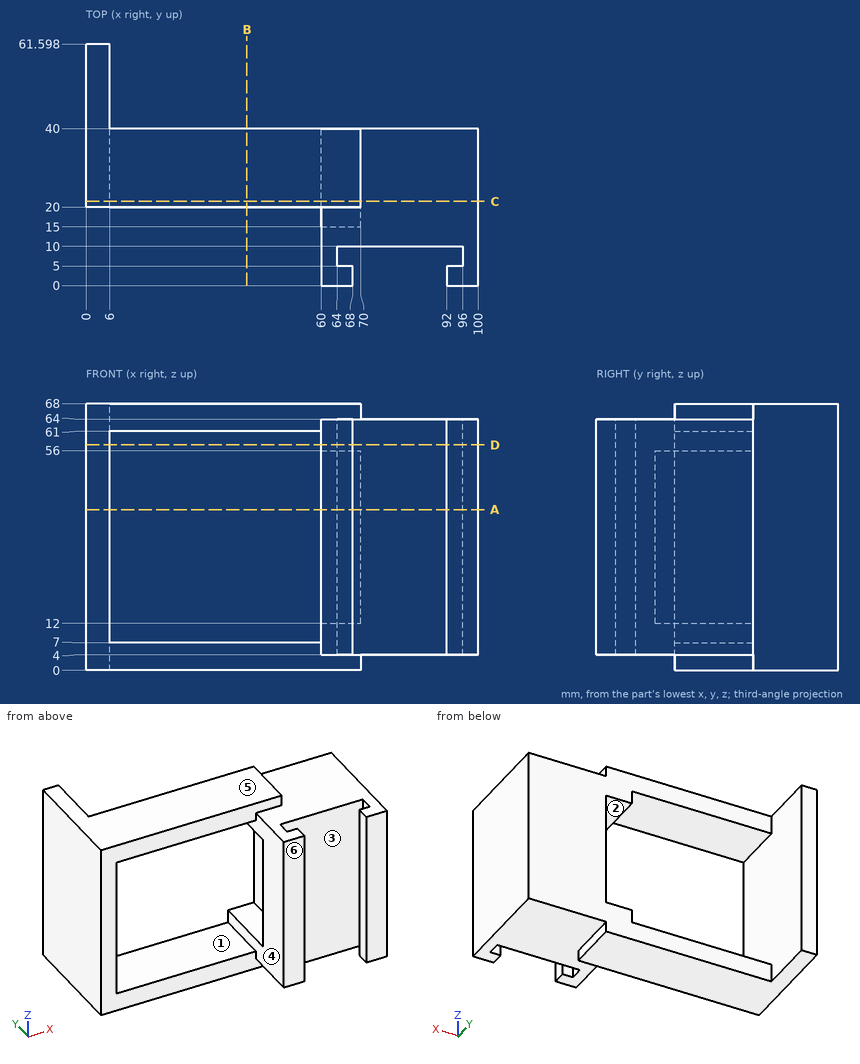
Source: three-view drawing plus pictorial views. Frame: mm from the lowest corner of the part. A direction names the side the tool comes from. Coordinates: 2 decimals unless noted, no trailing zeros. Order: outer loops, then holes, each group sorted by start corner. A loop starts at its lowest first (then second) coordinate and runs counter-clockwise, first axis right, second up. Notation, with made-up numbers: (47, 81.5) -> (93, 81.5) arc R21 ccw to (93, 100.5) -> close; hole circle Ø5 at (56, -39.5). An arc over 180 degrees is marked (long way). Write item = value, one per line.
(1) Pull-direction query (Z, two-part tool) for the marked faces 4, 5 and 6; classes: pulls with the +Z half, pulls with the -Z half, needs draft (parallel to the pull), parting line crosses it, or undercut.
Solved:
face_4 = undercut
face_5 = pulls with the +Z half
face_6 = needs draft
(2) Cut plane A-A on z = 41. Return loops of the section in (x, y), plus the area to 3 significant figures.
Solved:
outline = (0, 20) -> (6, 20) -> (6, 61.6) -> (0, 61.6) -> close; (60, 0) -> (68, 0) -> (68, 5) -> (64, 5) -> (64, 10) -> (96, 10) -> (96, 5) -> (92, 5) -> (92, 0) -> (100, 0) -> (100, 40) -> (70, 40) -> (70, 15) -> (60, 15) -> close
area = 1,320 mm²
(3) Pin query (flat end, axial travel): pin 1 Ø10 at (x, z) = (14, 7) entering from -Y; pin 2 Ø1.2 at (x, z) = (65.5, 42.5) entering from +Y; pin 3 Ø1.5 at (y, z) = (8, 41) entering from -X; pin 4 Ø20.5 at (x, z) = (34.5, 49.5) entering from +Y. Return the tip coordinate at first contact, or that it passes through.
Solved:
pin_1 = 20
pin_2 = 15
pin_3 = 60
pin_4 = through
(4) Access query for the marked faces 1, 2 and 3. Directions: +Z, -Z, +X, -X, +Y, -Y. A direction counts if a zero-diameter tool reaches every point of the face in a straight line with its end or side. Return the directions, or none.
Solved:
face_1 = +Y, -Y
face_2 = +Y
face_3 = +Z, -Z
(5) Cut plane C-C on y = 21.5. Return loops of the section in (x, z), plus the area to 3 significant figures.
Solved:
outline = (0, 0) -> (70, 0) -> (70, 4) -> (100, 4) -> (100, 64) -> (70, 64) -> (70, 68) -> (0, 68) -> close; hole (6, 7) -> (60, 7) -> (60, 12) -> (70, 12) -> (70, 56) -> (60, 56) -> (60, 61) -> (6, 61) -> close
area = 3,200 mm²
(6) Cut plane D-D on z = 57.5. Return loops of the section in (x, y), plus the area to 3 significant figures.
Solved:
outline = (0, 20) -> (6, 20) -> (6, 61.6) -> (0, 61.6) -> close; (60, 0) -> (68, 0) -> (68, 5) -> (64, 5) -> (64, 10) -> (96, 10) -> (96, 5) -> (92, 5) -> (92, 0) -> (100, 0) -> (100, 40) -> (60, 40) -> close
area = 1,570 mm²
(7) Cut plane B-B on x = 41. Return loops of the section in (y, z), plus the area to 3 significant figures.
Solved:
outline = (20, 0) -> (40, 0) -> (40, 7) -> (20, 7) -> close; (20, 61) -> (40, 61) -> (40, 68) -> (20, 68) -> close
area = 280 mm²
(8) Line query: line 1 (Z direction, x = 11, y = 27.5); line 2 (X direction, y = 7.5, z = 9); line 3 (X direction, y = 3, z = 17.5). Output: solid intervals per line, ascending.
Solved:
line_1 = 0 to 7, 61 to 68
line_2 = 60 to 64, 96 to 100
line_3 = 60 to 68, 92 to 100
